Answer from the drawing. Dimensions are ordinates in mm from the lowest x, y and z of the part. A direction names the side the tool comes from. Coordinates: 2 decimals unless noted, no trailing zeros. Write each loop counter-clockwise with the first axis right and the second up, starting at its lowest first coordinate (ties: lowest second). Pieces come first, ordered by that corner, then holes.
(1) Determine the mould class of the marked faces 3, 4 and 5 for opening direction Y: pulls with the +Y half, pulls with the -Y half, needs draft (parallel to the pull), parting line crosses it, or undercut.
(2) The part is cut by section C-C, the plane y = 24. Determine the outline of the cut face in (x, z) (1 decimal).
(3) The part is cut by section D-D, the plane x = 2.5. Determine the outline of the cut face in (y, z).
(4) Which of the six approach directions +Z, -Z, +X, -X, +Y, -Y give full straight-line access (tool end or side, diameter ignored) to the marked faces 1 and 2?
(5) Given pin 1 (2.5 mm diameter, centred on y = 20.75, z = 21.75, fed in from -X); pin 2 (13 mm diameter, centred on y = 20.75, z = 13.25, fed in from +X); pin 3 (3.5 mm diameter, centred on y = 20.75, z = 4.75, fed in from -X); pin 4 (5 mm diameter, centred on x = 10.75, z = 5.25, fed in from +Y), each flat-ended and moving along its own axis, determine where each tip first touches the part or whether it passes through.
(6) Straight lines are drawn through the part: line 1 along X through (y, z) = (0.8, 21.25); line 2 along Z through (x, y) = (24, 1); line 3 along X through (y, z) = (19, 8.75). For each, find the intervals that lie inside material, in ascending order.
(7) The part is cut by section B-B, the plane z = 13.25. Determine the outline of the cut face in (x, y).
(8) The part is cut by section A-A, the plane x = 17.8. Determine the outline of the cut face in (y, z), and give its area (3 significant figures).
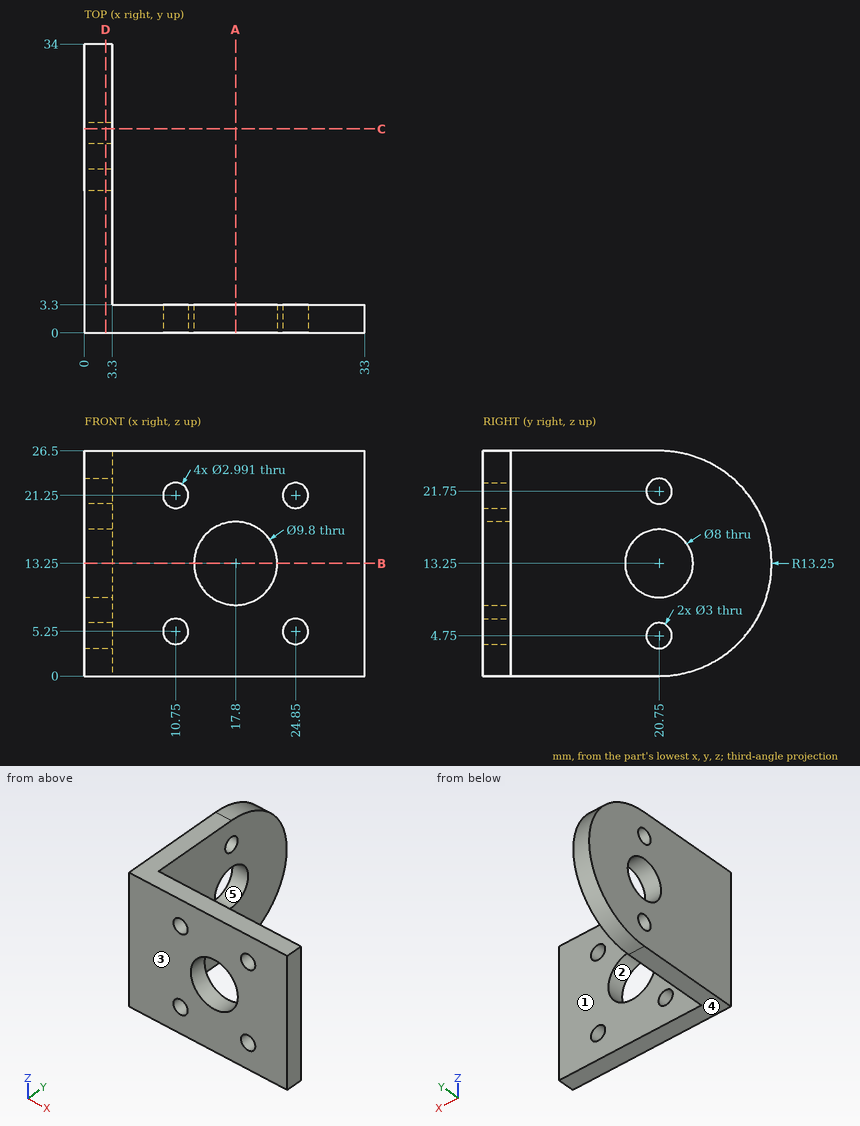
Computed:
1. face 3: pulls with the -Y half
1. face 4: needs draft
1. face 5: undercut
2. outline: (0, 0.4) - (3.3, 0.4) - (3.3, 10.9) - (0, 10.9) - close; (0, 15.6) - (3.3, 15.6) - (3.3, 26.1) - (0, 26.1) - close
3. outline: (0, 0) - (20.75, 0) arc R13.25 ccw to (20.75, 26.5) - (0, 26.5) - close; hole circle Ø8 at (20.75, 13.25); hole circle Ø3 at (20.75, 4.75); hole circle Ø3 at (20.75, 21.75)
4. face 1: +Z, -Z, +X, +Y
4. face 2: +Y, -Y
5. pin 1: passes through
5. pin 2: stops at x = 3.3
5. pin 3: stops at x = 0
5. pin 4: stops at y = 3.3
6. line 1: x = 0 to 9.25, 12.25 to 23.35, 26.35 to 33
6. line 2: z = 0 to 4.02, 6.48 to 20.02, 22.48 to 26.5
6. line 3: x = 0 to 3.3
7. outline: (0, 0) - (12.9, 0) - (12.9, 3.3) - (3.3, 3.3) - (3.3, 16.75) - (0, 16.75) - close; (0, 24.75) - (3.3, 24.75) - (3.3, 34) - (0, 34) - close; (22.7, 0) - (33, 0) - (33, 3.3) - (22.7, 3.3) - close
8. outline: (0, 0) - (3.3, 0) - (3.3, 8.35) - (0, 8.35) - close; (0, 18.15) - (3.3, 18.15) - (3.3, 26.5) - (0, 26.5) - close
8. area: 55.1 mm2
